from build123d import *

# Parameters (mm, degrees)
SALIENTE_EXTRUIR1_DEPTH = 3.175
CORTAR_EXTRUIR1_DEPTH   = 10


with BuildPart() as part:
    # Croquis1 → Saliente-Extruir1 (new body)
    with BuildSketch(Plane.XY):
        Polygon((-205.770387244, 310.6), (-205.770387244, -74.4), (-175.770387244, -74.4), (-175.770387244, -104.4), (444.229612756, -104.4), (444.229612756, -74.4), (474.229612756, -74.4), (474.229612756, 425.6), (444.229612756, 425.6), (444.229612756, 455.6), (-205.770387244, 455.6), (-205.770387244, 340.6), (-175.770387244, 340.6), (-175.770387244, 310.6), align=None)
    extrude(amount=SALIENTE_EXTRUIR1_DEPTH)

    # Croquis2 → Cortar-Extruir1 (cut)
    with BuildSketch(Plane.XY.offset(3.175)):
        Polygon((-205.770387244, 310.6), (-175.770387244, 310.6), (-175.770387244, 340.6), (-54.420387244, 340.6), (-54.420387244, 189.25), (-205.770387244, 189.25), align=None)
    extrude(amount=-CORTAR_EXTRUIR1_DEPTH, mode=Mode.SUBTRACT)


solid = part.part
Design review of the part built by this model. Coordinates are the model's own, in mm. Round coordinates to 2 decimals unless told otherwise and drop trailing zeros. Write each loop counter-clockwise with the first axis right and the second up, starting at its lowest first coordinate (ties: lowest second). Pieces come first, ordered by that corner, then holes.
Item 1: Consider section A-A on z = 1.4. Give the boundary of the cut face in (x, y).
Item 2: For pin 1 Ø1 at (y, z) = (240.5, 1) entering from -X; pin 2 Ø1 at (x, z) = (461.5, 1) entering from -Y; pin 3 Ø1 at (y, z) = (-92, 1.5) entering from -X, all flat-tipped, find the tip position at first contact; note any pin that passes through.
Item 3: Consider section B-B on y = 198.5. Give the boundary of the cut face in (x, z) (3 decimals).
Item 4: Wall thickness on L1, parallel to Y at x = -164.5, z = 2.5; L2, parallel to X at y = 299, z = 0.45: over which ranges is each line inside the solid? List them lowest first.
Check values:
1. outline: (-205.77, -74.4) - (-175.77, -74.4) - (-175.77, -104.4) - (444.23, -104.4) - (444.23, -74.4) - (474.23, -74.4) - (474.23, 425.6) - (444.23, 425.6) - (444.23, 455.6) - (-205.77, 455.6) - (-205.77, 340.6) - (-54.42, 340.6) - (-54.42, 189.25) - (-205.77, 189.25) - close
2. pin 1: stops at x = -54.42
2. pin 2: stops at y = -74.4
2. pin 3: stops at x = -175.77
3. outline: (-54.42, 0) - (474.23, 0) - (474.23, 3.175) - (-54.42, 3.175) - close
4. L1: y = -104.4 to 189.25, 340.6 to 455.6
4. L2: x = -54.42 to 474.23
